Input: part model. Units: mm. Frame: model coordinates. A direction names the side the tool comes from. Coordinates: 2 decimals unless noted, no trailing zeros. Write each loop counter-clockwise with the first axis right and the second up, starting at its lowest first coordinate (ties: lowest second). Pieces come first, ordered by that corner, then holes. Notation, with made-up numbers: M 39.25,-23 L 45.25,-23 A31 cw 45.25,2 Z; hole C 68,49 d11. An arc over 180 degrees is marked long. Use one line per item in the form item = value.
from build123d import *

# Parameters (mm, degrees)
BOSS_EXTRUDE1_DEPTH = 1.8
FILLET1_R           = 0.5


with BuildPart() as part:
    # Sketch1 → Boss-Extrude1 (new body)
    with BuildSketch(Plane.XY):
        with BuildLine():
            Line((0, 4.5), (0, 6.5))
            Line((0, 6.5), (6.1, 6.5))
            Line((6.1, 6.5), (6.1, 10.5))
            Line((6.1, 10.5), (10, 14.4))
            Line((10, 14.4), (10, 83.5))
            Line((10, 83.5), (16.4, 83.5))
            ThreePointArc((16.4, 83.5), (17.745328581, 80.945017946), (18.212299295, 78.095495067))
            Line((18.212299295, 78.095495067), (18.25, 49.5))
            Line((18.25, 49.5), (12, 49.5))
            Line((12, 49.5), (12, 37.18))
            add(Edge.make_bspline(
                [(12, 37.18), (12, 35.554764974), (12.5, 33.972282338), (12.5, 32.33)],
                knots=[0, 0, 0, 0, 1, 1, 1, 1], degree=3))
            Line((12.5, 32.33), (12.5, 3.07))
            ThreePointArc((12.5, 3.07), (11.600817818, 0.899182182), (9.43, 0))
            ThreePointArc((9.43, 0), (4.205660329, 1.182650422), (0, 4.5))
        make_face()
    extrude(amount=BOSS_EXTRUDE1_DEPTH)

    # Fillet1
    fillet1_edges = [part.edges().sort_by_distance(p)[0] for p in [
        (0, 6.5, 0.9),
        (6.1, 6.5, 0.9),
        (6.1, 10.5, 0.9),
        (10, 14.4, 0.9),
        (10, 83.5, 0.9),
        (18.25, 49.5, 0.9),
        (12, 49.5, 0.9),
    ]]
    fillet(fillet1_edges, radius=FILLET1_R)


solid = part.part
(1) Section query B-B on y = 23. Return the cut outline in (x, z).
Computed:
outline = M 10,0 L 12.5,0 L 12.5,1.8 L 10,1.8 Z
(2) Line query: probe 1 along X at (y, z) = (5, 0.85); probe 2 along Y at (x, z) = (14.5, 1.7); probe 3 along X at (y, z) = (7, 1). Output: solid intervals per line, ascending.
Computed:
probe_1 = 0 to 12.5
probe_2 = 49.5 to 83.5
probe_3 = 6.1 to 12.5
(3) Section query A-A on x = 13.75. Return the cut outline in (y, z), plus the area to 3 significant figures.
Computed:
outline = M 49.5,0 L 83.5,0 L 83.5,1.8 L 49.5,1.8 Z
area = 61.2 mm^2
(4) First-contact query: pin 1 Ø0.9 at (y, z) = (15.5, 0.5) entering from +X; pin 2 Ø0.5 at (y, z) = (33, 1) entering from -X; pin 3 Ø0.5 at (x, z) = (15, 0.5) entering from -Y. Flat tips, straight axial feed; report the tip coordinate or a pass-through.
Computed:
pin_1 = 12.5
pin_2 = 10
pin_3 = 49.5
(5) Pull-direction query (Y, two-part tool) for faces 4 (the flat face through (12, 43, 1)), 5 (the flat face through (0, 5, 1)), 6 (the flat face through (3, 6.5, 1)), 7 (the flat face through (15, 49.5, 1)); classes: pulls with the +Y half, pulls with the -Y half, needs draft (parallel to the pull), parting line crosses it, or undercut.
Computed:
face_4 = undercut
face_5 = needs draft
face_6 = pulls with the +Y half
face_7 = pulls with the -Y half
(6) Set-up query: faces 1 (the flat face through (10, 48, 1)), 2 (the flat face through (13, 83.5, 1)), 3 (the flat face through (12.5, 18, 1)). Return all of +Z, -Z, +X, -X, +Y, -Y with unobstructed straight access to the full face (end or side cutting, diameter ignored); none if empty.
Computed:
face_1 = +Z, -Z, -X, +Y
face_2 = +Z, -Z, +X, -X, +Y
face_3 = +Z, -Z, +X, -Y
